from build123d import *

# Parameters (mm, degrees)
F0_W      = 152.4
F0_H      = 152.4
F1_DEPTH  = 57.15
F2_R      = 5.08
F3_R      = 18.8722
F3_R_2    = 21.6916
F3_R_3    = 28.9306
F3_R_4    = 34.798
F3_R_5    = 15.2654
F3_R_6    = 24.9936
F4_DEPTH  = 50.8
F6_DEPTH  = 17.78
F8_DEPTH  = 50.8
F9_W      = 20.9688283503
F9_H      = 38.3084379137
F9_W_2    = 32.3605462909
F9_H_2    = 14.012824744
F9_W_3    = 35.6873329729
F9_H_3    = 6.3511356711
F9_W_4    = 32.1589261293
F9_W_5    = 20.5655843019
F9_H_4    = 34.1751612723
F10_DEPTH = 50.8
F12_DEPTH = 50.8
F13_W     = 32.2134252638
F13_H     = 13.5635472834
F14_DEPTH = 50.8


with BuildPart() as f1:
    # F0 (on Top) → F1 (new body)
    with BuildSketch(Plane.XY):
        Rectangle(F0_W, F0_H)
    extrude(amount=F1_DEPTH)

    # F2
    f2_edges = [f1.edges().sort_by_distance(p)[0] for p in [
        (-76.2, -76.2, 28.575),
        (76.2, -76.2, 28.575),
        (76.2, 76.2, 28.575),
        (-76.2, 76.2, 28.575),
        (76.2, 0, 57.15),
        (0, 76.2, 57.15),
        (-76.2, 0, 57.15),
        (0, -76.2, 57.15),
    ]]
    fillet(f2_edges, radius=F2_R)

    # F3 (on Top) → F4 (cut)
    with BuildSketch(Plane.XY):
        with Locations((-52.7972951531, -54.257504642)):
            Circle(F3_R)
        with Locations((-9.7686620429, -51.1906966567)):
            Circle(F3_R_2)
        with Locations((43.0286340415, -43.4057191014)):
            Circle(F3_R_3)
        with Locations((-39.074651897, 0)):
            Circle(F3_R_4)
        with Locations((11.8619473651, -10.1426448673)):
            Circle(F3_R_5)
        with Locations((47.4477931857, 12.9763726145)):
            Circle(F3_R_6)
    extrude(amount=F4_DEPTH, mode=Mode.SUBTRACT)

    # F5 (on Right) → F6 (cut, symmetric)
    with BuildSketch(Plane.YZ):
        with BuildLine():
            ThreePointArc((65.2309656143, 15.4240769103), (65.2771394427, 16.0320044258), (65.2925438309, 16.6414882988))
            ThreePointArc((65.2925438309, 16.6414882988), (53.3991094682, 28.7052683959), (41.1674231956, 16.9845848792))
            Line((41.1674231956, 16.9845848792), (65.2309656143, 16.9845848792))
            Line((65.2309656143, 16.9845848792), (65.2309656143, 15.4240769103))
        make_face()
        with BuildLine():
            Line((41.1674231956, 16.2983917184), (41.1674231956, 16.9845848792))
            ThreePointArc((41.1674231956, 16.9845848792), (41.1625438309, 16.6414882988), (41.1674231956, 16.2983917184))
        make_face()
        with BuildLine():
            Line((65.2309656143, 16.9845848792), (41.1674231956, 16.9845848792))
            Line((41.1674231956, 16.9845848792), (41.1674231956, 16.2983917184))
            ThreePointArc((41.1674231956, 16.2983917184), (52.7894681686, 4.584444104), (65.2309656143, 15.4240769103))
            Line((65.2309656143, 15.4240769103), (65.2309656143, 16.9845848792))
        make_face()
        with BuildLine():
            Line((65.2309656143, 0), (65.2309656143, 15.4240769103))
            ThreePointArc((65.2309656143, 15.4240769103), (52.7894681686, 4.584444104), (41.1674231956, 16.2983917184))
            Line((41.1674231956, 16.2983917184), (41.1674231956, 0))
            Line((41.1674231956, 0), (65.2309656143, 0))
        make_face()
    extrude(amount=F6_DEPTH, both=True, mode=Mode.SUBTRACT)

    # F7 (on Right) → F8 (cut, symmetric)
    with BuildSketch(Plane.YZ):
        with BuildLine():
            ThreePointArc((50.4576266435, 14.7510202975), (54.1037261363, 11.1856242821), (57.6962237544, 14.8050235584))
            ThreePointArc((57.6962237544, 14.8050235584), (57.6961230307, 14.8320259403), (57.6958208653, 14.8590268194))
            Line((57.6958208653, 14.8590268194), (50.4576266435, 14.8590268194))
            Line((50.4576266435, 14.8590268194), (50.4576266435, 14.7510202975))
        make_face()
        with BuildLine():
            ThreePointArc((57.6958208653, 14.8590268194), (57.6961230307, 14.8320259403), (57.6962237544, 14.8050235584))
            ThreePointArc((57.6962237544, 14.8050235584), (54.1037261363, 11.1856242821), (50.4576266435, 14.7510202975))
            Line((50.4576266435, 14.7510202975), (50.4576266435, -1.8991571851))
            Line((50.4576266435, -1.8991571851), (57.7001795173, -1.8991571851))
            Line((57.7001795173, -1.8991571851), (57.7001795173, 14.8590268194))
            Line((57.7001795173, 14.8590268194), (57.6958208653, 14.8590268194))
        make_face()
        with BuildLine():
            Line((50.4576266435, 14.8590268194), (57.6958208653, 14.8590268194))
            ThreePointArc((57.6958208653, 14.8590268194), (54.0767237544, 18.4245235584), (50.4576266435, 14.8590268194))
        make_face()
        with BuildLine():
            ThreePointArc((50.4576266435, 14.8590268194), (50.4572237544, 14.8050235584), (50.4576266435, 14.7510202975))
            Line((50.4576266435, 14.7510202975), (50.4576266435, 14.8590268194))
        make_face()
    extrude(amount=F8_DEPTH, both=True, mode=Mode.SUBTRACT)

    # F9 (on Top) → F10 (cut)
    with BuildSketch(Plane.XY):
        with Locations((-63.155984506, 53.8409817964)):
            Rectangle(F9_W, F9_H)
        with Locations((-35.3823676705, 65.9887883812)):
            Rectangle(F9_W_2, F9_H_2)
        with Locations((0.0529354438, 69.8196329176)):
            Rectangle(F9_W_3, F9_H_3)
        with Locations((35.0849926472, 65.9887883812)):
            Rectangle(F9_W_4, F9_H_2)
        with Locations((62.7577975392, 55.9076201171)):
            Rectangle(F9_W_5, F9_H_4)
    extrude(amount=F10_DEPTH, mode=Mode.SUBTRACT)

    # F11 (on Top) → F12 (cut)
    with BuildSketch(Plane.XY):
        Polygon((29.9793016165, 38.9572679996), (-17.8322065622, 38.9572679996), (-17.8322065622, 30.9886820614), (1.4958502725, 7.2524729185), (19.6370966733, 7.2524729185), (19.6370966733, 17.255589366), align=None)
    extrude(amount=F12_DEPTH, mode=Mode.SUBTRACT)

    # F13 (on Top) → F14 (cut)
    with BuildSketch(Plane.XY):
        with Locations((-35.3740798309, 42.3396099359)):
            Rectangle(F13_W, F13_H)
        Polygon((50.4153631628, 49.1213835776), (19.0496556461, 49.1213835776), (19.0496556461, 40.1355363429), (31.2568470836, 40.1355363429), (34.3086458743, 37.0837338269), (50.4153631628, 40.1355363429), align=None)
    extrude(amount=F14_DEPTH, mode=Mode.SUBTRACT)


solid = f1.part
Here's how the part is built. I have some questions about the finished solid (model axes, mm). A direction names the side the tool comes from. Coordinates: 2 decimals unless noted, no trailing zeros. Order: outer loops, then holes, each group sorted by start corner. A loop starts at its lowest first (then second) coordinate and runs counter-clockwise, first axis right, second up. Notation, with made-up numbers: M -25,64.25 L 32,64.25 A20 ccw 32,90.25 Z; hole C 70,-3.75 d7. An arc over 180 degrees is marked long. Answer as CSV lines item,"result".
Item 1: For pin 1 (6 mm diameter, centred on x = 47, y = 43, fed in from -Z), with a flat end and sliding along its axis, tell me the tip position at first contact or that it passes through.
Results found:
pin 1,"z = 50.8"
Item 2: We'd pull the mould along X, two halves only. Please class faces 1 (the face through (-1, 76.2, 26)), 2 (the face through (-74.751, 0.996, 55.622)), 3 (the face through (-66.69, -21.17, 25.04)): +X half, -X half, draft (parallel to the pull), parting line (faces both ways), or undercut.
Results found:
face 1,"draft"
face 2,"-X half"
face 3,"undercut"
Item 3: Imagine slicing it at C-C on z = 34.5. Give the number of separate pieces and of enclosed holes in the cut face, plus the area to 3 significant figures.
Results found:
separate pieces,"1"
enclosed holes,"14"
area,"7,020 mm2"
Item 4: On a 3-axis mill with a long thin cutter (end or side, diameter ignored), from which of +Z, -Z, +X, -X, +Y, -Y can I reach the whole of each face in a straight line? I mean faces 4 (the face through (0.996, -74.751, 55.622)), 5 (the face through (-17.791, 70, 25)). Say none if no direction works.
Results found:
face 4,"+Z, +X, -X, -Y"
face 5,"-Z"
Item 5: If I drill on line 1 (X direction, y = 46, z = 26.5) (3 decimals); line 2 (Y direction, x = 12, z = 43); line 3 (Y direction, x = -15, z = 48), over which ranges is the centre line in solid material (lowest first)?
Results found:
line 1,"-76.2 to -73.64, -52.672 to -51.481, -19.267 to 19.05, 50.415 to 52.475, 73.041 to 76.2"
line 2,"-76.2 to -25.41, 5.12 to 7.25, 38.96 to 66.64, 73 to 76.2"
line 3,"-76.2 to -72.24, -30.14 to -25.13, 25.13 to 27.51, 38.96 to 66.64, 73 to 76.2"
Item 6: Imagine slicing it at B-B on y = -60. Write out the boundary of the cut face in (x, z).
Results found:
outline,"M -76.2,0 L -70.77,0 L -70.77,50.8 L -34.82,50.8 L -34.82,0 L -29.59,0 L -29.59,50.8 L 10.05,50.8 L 10.05,0 L 19.33,0 L 19.33,50.8 L 66.73,50.8 L 66.73,0 L 76.2,0 L 76.2,52.07 A5.08 ccw 71.12,57.15 L -71.12,57.15 A5.08 ccw -76.2,52.07 Z"
